from build123d import *

# Parameters (mm, degrees)
SKETCH1_W               = 146.36
SKETCH1_H               = 101.6
BOSS_EXTRUDE1_DEPTH     = 3.18
CUT_EXTRUDE1_START      = -4.18
SKETCH2_W               = 3.18
SKETCH2_H               = 20
SKETCH2_W_2             = 13
SKETCH2_H_2             = 3
SKETCH2_W_3             = 2.82
SKETCH2_H_3             = 7
CUT_EXTRUDE1_DEPTH      = 5.18
CUT_EXTRUDE2_START      = -4.18
SKETCH3_W               = 63.305
SKETCH3_H               = 3.18
CUT_EXTRUDE2_DEPTH      = 5.18
SKETCH4_R               = 1.55
CUT_EXTRUDE3_DEPTH      = 1
CUT_EXTRUDE3_DEPTH_BACK = 4.18
SKETCH9_W               = 8
SKETCH9_H               = 8
CUT_EXTRUDE7_DEPTH      = 1
CUT_EXTRUDE7_DEPTH_BACK = 4.18
SKETCH8_R               = 1.4
CUT_EXTRUDE8_DEPTH      = 1
CUT_EXTRUDE8_DEPTH_BACK = 4.18
SKETCH12_R              = 1.4
CUT_EXTRUDE9_DEPTH      = 1
CUT_EXTRUDE9_DEPTH_BACK = 4.18


with BuildPart() as part:
    # Sketch1 → Boss-Extrude1 (new body)
    with BuildSketch(Plane.XY):
        Rectangle(SKETCH1_W, SKETCH1_H)
    extrude(amount=BOSS_EXTRUDE1_DEPTH)

    # Sketch2 → Cut-Extrude1 (cut)
    with BuildSketch(Plane.XY.offset(3.18).offset(CUT_EXTRUDE1_START)):
        with Locations((-71.59, 0)):
            Rectangle(SKETCH2_W, SKETCH2_H)
        with Locations((-66.68, 0)):
            Rectangle(SKETCH2_W_2, SKETCH2_H_2)
        with Locations((-64.59, 0)):
            Rectangle(SKETCH2_W_3, SKETCH2_H_3)
    cut_extrude1 = extrude(amount=CUT_EXTRUDE1_DEPTH, mode=Mode.SUBTRACT)

    # Mirror1: Cut-Extrude1 across plane
    add(cut_extrude1.mirror(Plane(origin=(0, 0, 0), x_dir=(0, 0, 1), z_dir=(1, 0, 0))), mode=Mode.SUBTRACT)

    # Sketch3 → Cut-Extrude2 (cut)
    with BuildSketch(Plane.XY.offset(3.18).offset(CUT_EXTRUDE2_START)):
        with Locations((-41.5275, -49.21)):
            Rectangle(SKETCH3_W, SKETCH3_H)
    cut_extrude2 = extrude(amount=CUT_EXTRUDE2_DEPTH, mode=Mode.SUBTRACT)

    # Mirror2: Cut-Extrude2 across plane
    add(cut_extrude2.mirror(Plane(origin=(0, 0, 0), x_dir=(0, 0, 1), z_dir=(1, 0, 0))), mode=Mode.SUBTRACT)

    # Sketch4 → Cut-Extrude3 (cut, two sides)
    with BuildSketch(Plane.XY.offset(3.18)) as cut_extrude3_sk:
        with Locations((0, -48.8)):
            Circle(SKETCH4_R)
    extrude(amount=CUT_EXTRUDE3_DEPTH, mode=Mode.SUBTRACT)
    extrude(cut_extrude3_sk.sketch, amount=-CUT_EXTRUDE3_DEPTH_BACK, mode=Mode.SUBTRACT)

    # Sketch9 → Cut-Extrude7 (cut, two sides)
    with BuildSketch(Plane(origin=(0, 0, 0), x_dir=(-1, 0, 0), z_dir=(0, 0, -1))) as cut_extrude7_sk:
        with Locations((14.920568418, -28.62)):
            Rectangle(SKETCH9_W, SKETCH9_H)
    extrude(amount=CUT_EXTRUDE7_DEPTH, mode=Mode.SUBTRACT)
    extrude(cut_extrude7_sk.sketch, amount=-CUT_EXTRUDE7_DEPTH_BACK, mode=Mode.SUBTRACT)

    # Sketch8 → Cut-Extrude8 (cut, two sides)
    with BuildSketch(Plane(origin=(0, 0, 0), x_dir=(-1, 0, 0), z_dir=(0, 0, -1))) as cut_extrude8_sk:
        with Locations((-5.716117592, -5.795275692)):
            Circle(SKETCH8_R)
        with Locations((-27.216117592, 7.954724308)):
            Circle(SKETCH8_R)
        with Locations((-27.216117592, -19.545275692)):
            Circle(SKETCH8_R)
    extrude(amount=CUT_EXTRUDE8_DEPTH, mode=Mode.SUBTRACT)
    extrude(cut_extrude8_sk.sketch, amount=-CUT_EXTRUDE8_DEPTH_BACK, mode=Mode.SUBTRACT)

    # Sketch12 → Cut-Extrude9 (cut, two sides)
    with BuildSketch(Plane(origin=(0, 0, 0), x_dir=(-1, 0, 0), z_dir=(0, 0, -1))) as cut_extrude9_sk:
        with Locations((19.68, 27.2)):
            Circle(SKETCH12_R)
        with Locations((33.43, 5.7)):
            Circle(SKETCH12_R)
        with Locations((47.18, 27.2)):
            Circle(SKETCH12_R)
    extrude(amount=CUT_EXTRUDE9_DEPTH, mode=Mode.SUBTRACT)
    extrude(cut_extrude9_sk.sketch, amount=-CUT_EXTRUDE9_DEPTH_BACK, mode=Mode.SUBTRACT)


solid = part.part
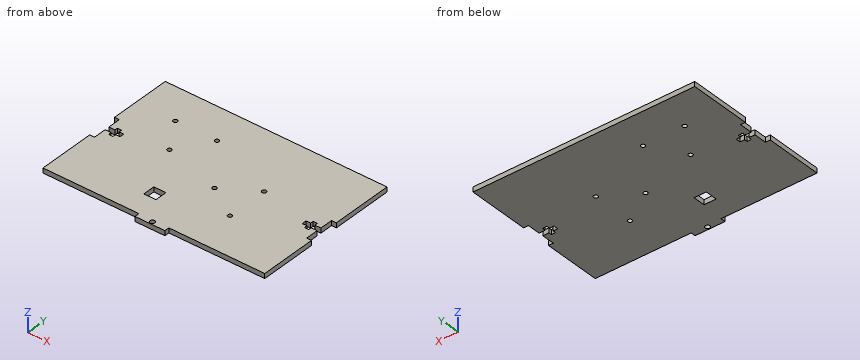
Geometry check sheet. Reference: the model listing, model coordinates, mm. Give positions to 0.01 mm unless a question says otherwise; leave off trailing zeros. Write each loop counter-clockwise with the first axis right and the second up, starting at its lowest first coordinate (ties: lowest second). Pieces come first, ordered by that corner, then holes. Notation, with made-up numbers: M 8.5,10 L 21.5,10 A15 cw 21.5,24 Z; hole C -21.5,-32 d4. An arc over 180 degrees is marked long. Answer as CSV lines item,"result". Start each with the question number.
Q1. Go/stop test with flat-tipped pins: pin 1 (1.6 mm diameter, centred on x = 47, z = 1.5, fed in from -Y); pin 2 (1 mm diameter, centred on y = -2.5, z = 1, fed in from +X); pin 3 (1.7 mm diameter, centred on x = 27.22, y = -19.55, fed in from +Z); pin 4 (1.6 mm diameter, centred on y = -50, z = 1.5, fed in from +X) (3 decimals). Record where each tip stops, or that it passes through.
Q2. Section check B-B, the plane z = 0.9. Give the number of separate pieces and of enclosed holes in the cut face, then the cut area to 3 significant figures.
Q3. Material ranges on L1, parallel to Y at x = -47.18, z = 1.1; L2, parallel to Y at x = -64, z = 2.7; L3, parallel to Y at x = -31, z = 2.7, recorded low to high.
Q4. Section check A-A, the plane x = 0. Record the cut outline in (y, z).
Q5. Section check C-C, the plane x = -54. Record the cut outline in (y, z).
Geometry says:
1,pin 1,"y = -47.62"
1,pin 2,"x = 70"
1,pin 3,"through"
1,pin 4,"x = 9.875"
2,separate pieces,"1"
2,enclosed holes,"8"
2,area,"14,200 mm^2"
3,L1,"-47.62 to 25.8, 28.6 to 50.8"
3,L2,"-47.62 to -3.5, 3.5 to 50.8"
3,L3,"-47.62 to 50.8"
4,outline,"M -50.8,0 L -50.35,0 L -50.35,3.18 L -50.8,3.18 Z; M -47.25,0 L 50.8,0 L 50.8,3.18 L -47.25,3.18 Z"
5,outline,"M -47.62,0 L 50.8,0 L 50.8,3.18 L -47.62,3.18 Z"
